Part model, mm, in its own coordinate system. A direction names the side the tool comes from. Round coordinates to 2 decimals unless told otherwise and drop trailing zeros. Write each loop counter-clockwise with the first axis right and the second up, starting at its lowest first coordinate (ties: lowest second). Pieces come first, ordered by that corner, then holes. Notation, with made-up numbers: M -12.5,49.5 L 42.5,49.5 A32 ccw 42.5,79.5 Z; hole C 78.25,-25 d9. An arc over 180 degrees is marked long. Use one line per item in the form item = value. Start each with the question number.
Item 1: Cut at A-A, the plane x = -12.7. Give the cut face in (y, z).
Item 2: Which spindle directions (+Z, -Z, +X, -X, +Y, -Y) get a long thin tool onto all of the face, cutting with end or side? Do faces 1 (the face through (-13.41, -61.56, 72)), 2 (the face through (-55, -61, 140.462)). Say none if no direction does.
Item 3: Cut at B-B, the plane y = -63. Give the cut face in (x, z).
Item 4: Flat gauge pins, fed straight in: pin 1 Ø10.5 at (x, z) = (-12.7, 62.484) entering from -Y; pin 2 Ø1 at (y, z) = (-57.5, 115) entering from -X. Where does each tip first touch, or does it go through?
Item 5: Cut at C-C, the plane z = 125. Give the cut face in (x, y), then the cut area to 3 significant figures.
Item 6: Cut at D-D, the plane x = -65.5. Give the cut face in (y, z), then the cut area to 3 significant figures.
Item 7: Mould opens along Z. For faces 3 (the face through (12.28, -61.56, 91.12)), 4 (the face through (-29.718, -62, 92)), 5 (the face through (-25, -61, 146.812)), 6 (the face through (0, -61, 45.212)) say: +Z half, -Z half, draft (parallel to the pull), parting line (faces both ways), or undercut.
Item 8: Probe L1, parallel to Z at x = 12.7, y = -59; L2, parallel to X at y = -66.75, z = 76; L3, parallel to X at y = -64, z = 78. List the from-to ranges inside material, lowest first.
from build123d import *

# Parameters (mm, degrees)
SKETCH024_W        = 59.436
SKETCH024_H        = 12.7
PAD003003_DEPTH    = 101.6
SKETCH026_R        = 3.2639
POCKET001003_DEPTH = 12.701
SKETCH025_W        = 12.7
SKETCH025_H        = 6.35
PAD003004_DEPTH    = 50.8


with BuildPart() as part:
    # Sketch024 → Pad003003 (new body)
    with BuildSketch(Plane.XY.offset(45.212)):
        with Locations((0, -61.468)):
            Rectangle(SKETCH024_W, SKETCH024_H)
    extrude(amount=PAD003003_DEPTH)

    # Sketch026 (on Face1 of Pad003003) → Pocket001003 (cut, through all)
    with BuildSketch(Plane(origin=(0, -67.818, 45.212), x_dir=(1, 0, 0), z_dir=(0, -1, 0))):
        with Locations((-12.7, 17.272)):
            Circle(SKETCH026_R)
        with Locations((-12.7, 29.972)):
            Circle(SKETCH026_R)
        with Locations((-12.7, 42.672)):
            Circle(SKETCH026_R)
        with Locations((12.7, 17.272)):
            Circle(SKETCH026_R)
        with Locations((12.7, 29.972)):
            Circle(SKETCH026_R)
        with Locations((12.7, 42.672)):
            Circle(SKETCH026_R)
    extrude(amount=-POCKET001003_DEPTH, mode=Mode.SUBTRACT)

    # Sketch025 (on Face5 of Pocket001003) → Pad003004 (join)
    with BuildSketch(Plane(origin=(-29.718, 0, 45.212), x_dir=(0, -1, 0), z_dir=(-1, 0, 0))):
        with Locations((61.468, 98.425)):
            Rectangle(SKETCH025_W, SKETCH025_H)
    extrude(amount=PAD003004_DEPTH)


solid = part.part
Model answer:
q1.outline = M -67.82,45.21 L -55.12,45.21 L -55.12,59.22 L -67.82,59.22 Z; M -67.82,65.75 L -55.12,65.75 L -55.12,71.92 L -67.82,71.92 Z; M -67.82,78.45 L -55.12,78.45 L -55.12,84.62 L -67.82,84.62 Z; M -67.82,91.15 L -55.12,91.15 L -55.12,146.81 L -67.82,146.81 Z
q2.face_1 = +Y, -Y
q2.face_2 = -Z, -X, +Y, -Y
q3.outline = M -80.52,140.46 L -29.72,140.46 L -29.72,45.21 L 29.72,45.21 L 29.72,146.81 L -80.52,146.81 Z; hole C -12.7,62.48 d6.53; hole C -12.7,75.18 d6.53; hole C -12.7,87.88 d6.53; hole C 12.7,62.48 d6.53; hole C 12.7,75.18 d6.53; hole C 12.7,87.88 d6.53
q4.pin_1 = -67.82
q4.pin_2 = -29.72
q5.outline = M -29.72,-67.82 L 29.72,-67.82 L 29.72,-55.12 L -29.72,-55.12 Z
q5.area = 755 mm²
q6.outline = M -67.82,140.46 L -55.12,140.46 L -55.12,146.81 L -67.82,146.81 Z
q6.area = 80.6 mm²
q7.face_3 = undercut
q7.face_4 = draft
q7.face_5 = +Z half
q7.face_6 = -Z half
q8.L1 = 45.21 to 59.22, 65.75 to 71.92, 78.45 to 84.62, 91.15 to 146.81
q8.L2 = -29.72 to -15.86, -9.54 to 9.54, 15.86 to 29.72
q8.L3 = -29.72 to -14.35, -11.05 to 11.05, 14.35 to 29.72
